The model under review builds one solid part; all positions refer to its coordinate system, in mm. A direction names the side the tool comes from. Give positions to 0.01 mm unless a question says otherwise; leave off trailing zeros. Loops run counter-clockwise (first coordinate to the right, second up) from the corner with the lowest first, then second, coordinate; pieces in that order, holes last. Notation, with made-up numbers: (15.5, 75) - (33.5, 75) arc R17 ccw to (33.5, 101) - close; hole circle Ø2 at (39.25, -24.5). An arc over 180 degrees is marked (long way). Return JSON: item names as keys, results as strings. Group by question number.
```python
from build123d import *

# Parameters (mm, degrees)
BOSS_EXTRUDE1_DEPTH      = 10
BOSS_EXTRUDE1_DEPTH_BACK = 15
SKETCH1_W                = 1016
SKETCH1_H                = 304.8
SKETCH1_W_2              = 996
SKETCH1_H_2              = 284.8
BOSS_EXTRUDE2_DEPTH      = 10
BOSS_EXTRUDE2_DEPTH_BACK = 15
BOSS_EXTRUDE3_DEPTH      = 152.4
BOSS_EXTRUDE3_DEPTH_BACK = 152.4
SKETCH4_W                = 507.049279033
SKETCH4_H                = 40
BOSS_EXTRUDE7_DEPTH      = 5
SKETCH5_W                = 284.8
SKETCH5_H                = 234
CUT_EXTRUDE1_DEPTH       = 15
SKETCH6_W                = 284.8
SKETCH6_H                = 234
CUT_EXTRUDE2_DEPTH       = 15
BOSS_EXTRUDE8_DEPTH      = 304.8
BOSS_EXTRUDE9_DEPTH      = 5
BOSS_EXTRUDE10_DEPTH     = 5


with BuildPart() as part:
    # Sketch1 → Boss-Extrude1 (new, two sides: drawn at the far end of the back side and taken through both)
    with BuildSketch(Plane(origin=(0, 0, 0), x_dir=(1, 0, 0), z_dir=(0, 1, 0)).offset(-BOSS_EXTRUDE1_DEPTH_BACK)):
        Rectangle(SKETCH1_W, SKETCH1_H)
        Rectangle(SKETCH1_W_2, SKETCH1_H_2, mode=Mode.SUBTRACT)
    extrude(amount=BOSS_EXTRUDE1_DEPTH + BOSS_EXTRUDE1_DEPTH_BACK)

    # Sketch2 → Boss-Extrude2 (add, two sides: drawn at the far end of the back side and taken through both)
    with BuildSketch(Plane(origin=(0, 0, 0), x_dir=(1, 0, 0), z_dir=(0, 1, 0)).offset(-BOSS_EXTRUDE2_DEPTH_BACK)):
        with BuildLine():
            Line((-498, 20), (-30, 20))
            ThreePointArc((-30, 20), (-22.928932188, 22.928932188), (-20, 30))
            Line((-20, 30), (-20, 142.4))
            Line((-20, 142.4), (-10, 142.4))
            Line((-10, 142.4), (-10, 20))
            Line((-10, 20), (-10, 10))
            Line((-10, 10), (-498, 10))
            Line((-498, 10), (-498, 20))
        make_face()
        with BuildLine():
            Line((498, 20), (498, 10))
            Line((498, 10), (10, 10))
            Line((10, 10), (10, 20))
            Line((10, 20), (10, 142.4))
            Line((10, 142.4), (20, 142.4))
            Line((20, 142.4), (20, 30))
            ThreePointArc((20, 30), (22.928932188, 22.928932188), (30, 20))
            Line((30, 20), (498, 20))
        make_face()
        with BuildLine():
            Line((-498, -10), (-10, -10))
            Line((-10, -10), (-10, -20))
            Line((-10, -20), (-10, -142.4))
            Line((-10, -142.4), (-20, -142.4))
            Line((-20, -142.4), (-20, -30))
            ThreePointArc((-20, -30), (-22.928932188, -22.928932188), (-30, -20))
            Line((-30, -20), (-498, -20))
            Line((-498, -20), (-498, -10))
        make_face()
        with BuildLine():
            Line((30, -20), (498, -20))
            Line((498, -20), (498, -10))
            Line((498, -10), (10, -10))
            Line((10, -10), (10, -20))
            Line((10, -20), (10, -142.4))
            Line((10, -142.4), (20, -142.4))
            Line((20, -142.4), (20, -30))
            ThreePointArc((20, -30), (22.928932188, -22.928932188), (30, -20))
        make_face()
    extrude(amount=BOSS_EXTRUDE2_DEPTH + BOSS_EXTRUDE2_DEPTH_BACK)

    # Sketch3 → Boss-Extrude3 (add, two sides: drawn at the far end of the back side and taken through both)
    with BuildSketch(Plane.XY.offset(-BOSS_EXTRUDE3_DEPTH_BACK)):
        Polygon((-508, 10), (-508, 264), (-254, 10), (-261.071067812, 10), (-503, 251.928932188), (-503, 10), align=None)
        Polygon((261.071067812, 10), (254, 10), (508, 264), (508, 10), (503, 10), (503, 251.928932188), align=None)
    extrude(amount=BOSS_EXTRUDE3_DEPTH + BOSS_EXTRUDE3_DEPTH_BACK)

    # Sketch4 → Boss-Extrude7 (add)
    with BuildSketch(Plane(origin=(0, 10, 0), x_dir=(1, 0, 0), z_dir=(0, 1, 0))):
        with Locations((-0.42499269, 0)):
            Rectangle(SKETCH4_W, SKETCH4_H)
    extrude(amount=BOSS_EXTRUDE7_DEPTH)

    # Sketch5 → Cut-Extrude1 (cut)
    with BuildSketch(Plane(origin=(508, 0, 0), x_dir=(0, 0, -1), z_dir=(1, 0, 0))):
        with Locations((0, 127)):
            Rectangle(SKETCH5_W, SKETCH5_H)
    extrude(amount=-CUT_EXTRUDE1_DEPTH, mode=Mode.SUBTRACT)

    # Sketch6 → Cut-Extrude2 (cut)
    with BuildSketch(Plane.ZY.offset(508)):
        with Locations((0, 127)):
            Rectangle(SKETCH6_W, SKETCH6_H)
    extrude(amount=-CUT_EXTRUDE2_DEPTH, mode=Mode.SUBTRACT)

    # Sketch7 → Boss-Extrude8 (add)
    with BuildSketch(Plane(origin=(0, 0, -152.4), x_dir=(-1, 0, 0), z_dir=(0, 0, -1))):
        Polygon((-49.38581657, 10), (-9.847908285, 49.537908285), (10.152091715, 49.537908285), (49.69, 10), align=None)
    extrude(amount=-BOSS_EXTRUDE8_DEPTH)

    # Sketch8 → Boss-Extrude9 (add)
    with BuildSketch(Plane.XY.offset(152.4)):
        Polygon((-508, 264), (508, 264), (254, 10), (-254, 10), align=None)
    extrude(amount=-BOSS_EXTRUDE9_DEPTH)

    # Sketch9 → Boss-Extrude10 (add)
    with BuildSketch(Plane(origin=(0, 0, -152.4), x_dir=(-1, 0, 0), z_dir=(0, 0, -1))):
        Polygon((-508, 264), (508, 264), (254, 10), (-254, 10), align=None)
    extrude(amount=-BOSS_EXTRUDE10_DEPTH)


solid = part.part
```
1) Draft analysis for pull direction X (two halves, no side actions). For faces 4 (the face through (-10, -3, -77)), 5 (the face through (34, 10, 80)), 6 (the face through (-7, 126, -152.4)), state which applies: +X half, -X half, draft (parallel to the pull), parting line (faces both ways), or undercut.
2) We need section C-C, the plane y = 140. Write out the cut boundary in (x, z), plus the area to 3 significant figures.
3) We need section D-D, the plane z = 41. Count the separate pieces of the cut face and the enclosed holes in it, plus the area to 3 significant figures.
4) For pin 1 Ø1.7 at (y, z) = (242.5, 4.5) entering from +X; pin 2 Ø2 at (x, z) = (257, 110) entering from -Y; pin 3 Ø2.5 at (x, z) = (135, -146) entering from +Y, all flat-tipped, find the tip position at first contact; note any pin that passes through.
5) We need section B-B, the plane y = 76. Write out the cut boundary in (x, z), plus the area to 3 significant figures.
6) Tool access review of faces 1 (the face through (-251, -3, -10)), 2 (the face through (0, 49.538, -2)), 3 (the face through (-403, 10, 11)): name each direction out of +Z, -Z, +X, -X, +Y, -Y from which nothing blocks a thin tool from reaching the whole face with its end or side.
7) We need section A-A, the plane x = -63.5. Write out the cut boundary in (y, z).
8) To check wall thickness, follow line 1 (Z direction, x = -402.5, y = -4); line 2 (Z direction, x = -421, y = 180); line 3 (X direction, y = 42, z = -0.5). State the ranges of each line that lie inside material, in increasing order.
Findings:
{
 "1": {"face 4": "undercut", "face 5": "undercut", "face 6": "draft"},
 "2": {"outline": "(-508, -152.4) - (-503, -152.4) - (-503, -142.4) - (-508, -142.4) - close; (-508, 142.4) - (-503, 142.4) - (-503, 152.4) - (-508, 152.4) - close; (-391.07, -152.4) - (391.07, -152.4) - (391.07, 152.4) - (-391.07, 152.4) - close; (503, -152.4) - (508, -152.4) - (508, -142.4) - (503, -142.4) - close; (503, 142.4) - (508, 142.4) - (508, 152.4) - (503, 152.4) - close; hole (-384, -147.4) - (384, -147.4) - (384, 147.4) - (-384, 147.4) - close", "area": "12,200 mm^2"},
 "3": {"separate pieces": "5", "enclosed holes": "0", "area": "7,000 mm^2"},
 "4": {"pin 1": "stops at x = 493", "pin 2": "stops at y = 10", "pin 3": "stops at y = 10"},
 "5": {"outline": "(-508, -152.4) - (-503, -152.4) - (-503, -142.4) - (-508, -142.4) - close; (-508, 142.4) - (-503, 142.4) - (-503, 152.4) - (-508, 152.4) - close; (-327.07, -152.4) - (327.07, -152.4) - (327.07, 152.4) - (-327.07, 152.4) - close; (503, -152.4) - (508, -152.4) - (508, -142.4) - (503, -142.4) - close; (503, 142.4) - (508, 142.4) - (508, 152.4) - (503, 152.4) - close; hole (-320, -147.4) - (320, -147.4) - (320, 147.4) - (-320, 147.4) - close", "area": "10,900 mm^2"},
 "6": {"face 1": "-Y", "face 2": "+Y", "face 3": "none"},
 "7": {"outline": "(-15, -152.4) - (264, -152.4) - (264, -147.4) - (10, -147.4) - (10, -142.4) - (-15, -142.4) - close; (-15, -20) - (15, -20) - (15, 20) - (-15, 20) - (-15, 10) - (10, 10) - (10, -10) - (-15, -10) - close; (-15, 142.4) - (10, 142.4) - (10, 147.4) - (264, 147.4) - (264, 152.4) - (-15, 152.4) - close"},
 "8": {"line 1": "z = -152.4 to -142.4, -20 to -10, 10 to 20, 142.4 to 152.4", "line 2": "z = -152.4 to -147.4, 147.4 to 152.4", "line 3": "x = -293.07 to -286, -17.69 to 17.39, 286 to 293.07"}
}
